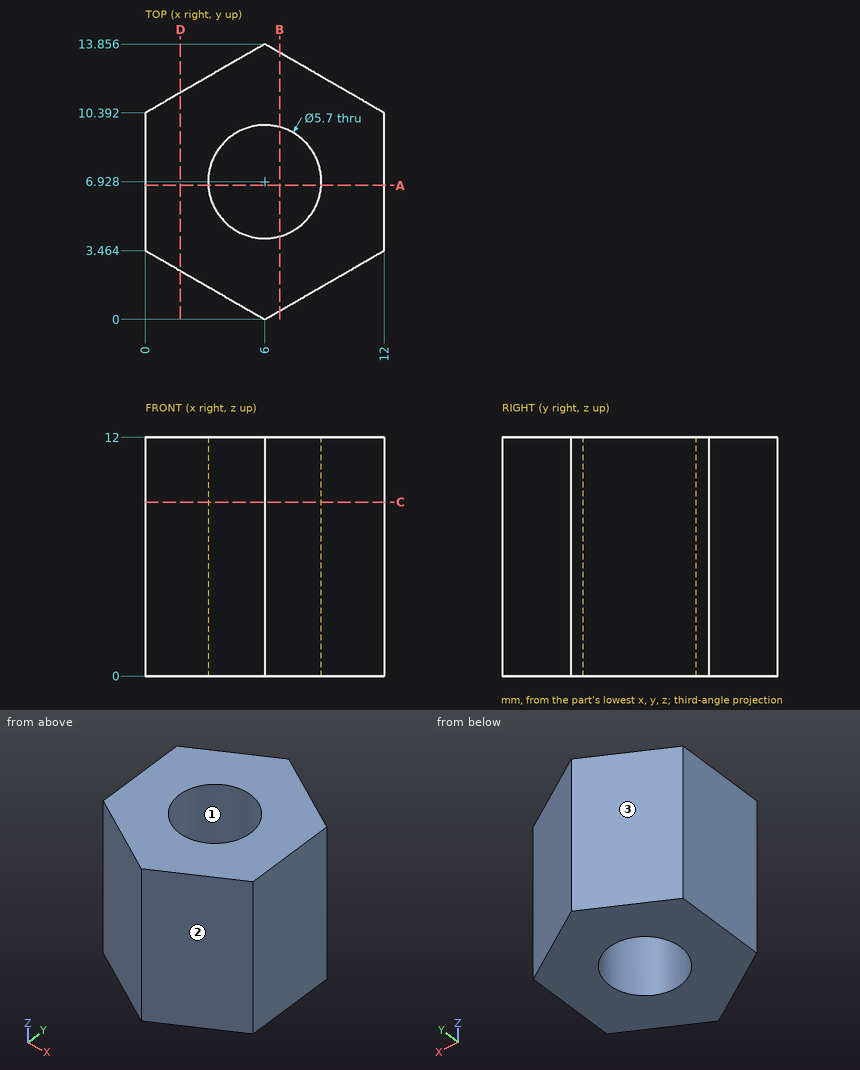
Source: three-view drawing plus pictorial views. Frame: mm from the lowest corner of the part. Round coordinates to 2 decimals unless told otherwise and drop trailing zeros. Write each loop counter-clockwise with the first axis right and the second up, starting at its lowest first coordinate (ties: lowest second). Pieces come first, ordered by that corner, then holes. Notation, with made-up numbers: M -19,22 L 22,22 A9 ccw 22,34 Z; hole C 89.5,48 d9. An arc over 180 degrees is marked long. Use CSV: the item, a comma, the result in double quotes. Start each with the question number.
Q1. Cut plane C-C on z = 8.75. Output: boundary loops of the cut face in (x, y).
Q2. Cut plane D-D on x = 1.75. Output: boundary loops of the cut face in (y, z), plus the area to 3 significant figures.
Q3. Pull-direction query (Y, two-part tool) for the marked faces 1, 2 and 3; classes: +Y half, -Y half, draft (parallel to the pull), parting line (faces both ways), or undercut.
Q4. Line query: line 1 (Y direction, x = 5.5, z = 1.5) (1 decimal); line 2 (X direction, y = 5.5, z = 0.5) (1 decimal); line 3 (X direction, y = 6.5, z = 0.5). Output: solid intervals per line, ascending. Write a range as from..to.
Q5. Cut plane B-B on x = 6.75. Output: boundary loops of the cut face in (y, z).
Q6. First-contact query: P1, Ø3, axis at x = 4, z = 10.5, coming from the -Y side; P2, Ø1, axis at y = 10.5, z = 10, coming from the -X side; P3, Ø5, axis at x = 2, z = 5.5, coming from the -Y side (1 decimal); P4, Ø1.5, axis at y = 2, z = 5, coming from the -X side (1 decimal). Flat tips, straight axial feed; report the tip coordinate or a pass-through.
Q7. Cut plane A-A on y = 6.75. Output: boundary loops of the cut face in (x, z) (1 decimal).
Results found:
1,outline,"M 0,3.46 L 6,0 L 12,3.46 L 12,10.39 L 6,13.86 L 0,10.39 Z; hole C 6,6.93 d5.7"
2,outline,"M 2.45,0 L 11.4,0 L 11.4,12 L 2.45,12 Z"
2,area,"107 mm^2"
3,face 1,"undercut"
3,face 2,"-Y half"
3,face 3,"+Y half"
4,line 1,"0.3..4.1, 9.7..13.6"
4,line 2,"0..3.5, 8.5..12"
4,line 3,"0..3.18, 8.82..12"
5,outline,"M 0.43,0 L 4.18,0 L 4.18,12 L 0.43,12 Z; M 9.68,0 L 13.42,0 L 13.42,12 L 9.68,12 Z"
6,P1,"y = 0.29"
6,P2,"x = 0"
6,P3,"y = 0.9"
6,P4,"x = 1.2"
7,outline,"M 0,0 L 3.2,0 L 3.2,12 L 0,12 Z; M 8.8,0 L 12,0 L 12,12 L 8.8,12 Z"
